Work out the finished part from the listing and answer in its coordinate system (mm). Coordinates: 2 decimals unless noted, no trailing zeros. Order: outer loops, then holes, each group sorted by start corner. A loop starts at its lowest first (then second) coordinate and runs counter-clockwise, first axis right, second up. Notation, with made-up numbers: (-31, 76) -> (4, 76) arc R37 cw to (4, 113) -> close; hole circle Ø5 at (89.25, 8). An arc over 180 degrees is marked (long way). Write item = value, one per line. Start each with the question number.
Q1. The part is cut by section D-D, the plane z = 1.75. Determine the outline of the cut face in (x, y).
Q2. The part is cut by section A-A, the plane z = -8. Determine the outline of the cut face in (x, y) (1 decimal).
Q3. Straight lines are drawn through the part: L1, parallel to Y at x = 0, z = 0.1; L2, parallel to Z at x = -15, y = -25 (3 decimals); L3, parallel to Y at x = 0, z = 0.4. For each, find the intervals that lie inside material, in ascending order. Write a range as from..to.
Q4. Flat-ended cylindrical pins translate along their axes: pin 1 (4 mm diameter, centred on x = -12.5, y = -10, fed in from -Z); pin 2 (4 mm diameter, centred on x = -25.4, y = 0, fed in from +Z); pin 3 (6 mm diameter, centred on x = 0, y = -25.4, fed in from +Z); pin 4 (1 mm diameter, centred on y = 11, z = 1, fed in from +X). Find the tip coordinate at first contact, or state that the pin passes through.
Q5. For a pull along X with two mould halves and no side action, classify faces 1 (the cylindrical face through (-3.78, 2.9, -6.27)), 2 (the cylindrical face through (0.487, -27.594, 0.254)), 3 (the flat face through (2, 2, -12.7)) as +X half, -X half, draft (parallel to the pull), parting line (faces both ways), or undercut.
Q6. The part is cut by section B-B, the plane y = 0. Count the separate pieces of the cut face and the enclosed holes in it, plus the area to 3 significant figures.
```python
from build123d import *

# Parameters (mm, degrees)
F0_R           = 31.75
F1_DEPTH       = 3.175
F2_R           = 4.7625
F3_DEPTH       = 12.7
F5_D           = 4.4958
F5_CSINK_D     = 9.1186
F5_CSINK_ANGLE = 82
F6_R           = 1.9812
F7_DEPTH       = 15.876
F8_SIZE        = 0.508


with BuildPart() as f1:
    # F0 (on Top) → F1 (new body)
    with BuildSketch(Plane.XY):
        Circle(F0_R)
    extrude(amount=F1_DEPTH)

    # F2 (on face) → F3 (join)
    with BuildSketch(Plane(origin=(0, 0, 0), x_dir=(1, 0, 0), z_dir=(0, 0, -1))):
        Circle(F2_R)
    extrude(amount=F3_DEPTH)

    # F5 (through all)
    with Locations(Plane.XY.offset(3.175)):
        with Locations((-25.4, 0), (0, 25.4), (25.4, 0), (0, -25.4)):
            CounterSinkHole(F5_D / 2, F5_CSINK_D / 2, counter_sink_angle=F5_CSINK_ANGLE)

    # F6 (on face) → F7 (cut, through all)
    with BuildSketch(Plane.XY.offset(3.175)):
        Circle(F6_R)
    extrude(amount=-F7_DEPTH, mode=Mode.SUBTRACT)

    # F8
    f8_edges = [f1.edges().sort_by_distance(p)[0] for p in [
        (-31.75, 0, 3.175),
        (-1.9812, 0, 3.175),
        (-31.75, 0, 0),
        (-4.7625, 0, -12.7),
        (-1.9812, 0, -12.7),
        (-4.7625, 0, 0),
    ]]
    chamfer(f8_edges, length=F8_SIZE)


solid = f1.part
```
Model answer:
q1.outline = circle Ø63.5 at (0, 0); hole circle Ø6.64 at (-25.4, 0); hole circle Ø6.64 at (0, -25.4); hole circle Ø6.64 at (0, 25.4); hole circle Ø3.96 at (0, 0); hole circle Ø6.64 at (25.4, 0)
q2.outline = circle Ø9.5 at (0, 0); hole circle Ø4 at (0, 0)
q3.L1 = -31.34..-27.65, -23.15..-1.98, 1.98..23.15, 27.65..31.34
q3.L2 = 0..3.175
q3.L3 = -31.64..-27.65, -23.15..-1.98, 1.98..23.15, 27.65..31.64
q4.pin_1 = 0
q4.pin_2 = through
q4.pin_3 = 1.38
q4.pin_4 = 29.96
q5.face_1 = parting line
q5.face_2 = undercut
q5.face_3 = draft
q6.separate_pieces = 4
q6.enclosed_holes = 0
q6.area = 218 mm2
